```python
from build123d import *

# Parameters (mm, degrees)
SKETCH1_R           = 3.175
BOSS_EXTRUDE1_DEPTH = 57.15


with BuildPart() as part:
    # Sketch1 → Boss-Extrude1 (new body)
    with BuildSketch(Plane.XZ.offset(57.15)):
        with BuildLine():
            Line((-4.682174209, -4.59023638), (-3.666174209, -6.35))
            Line((-3.666174209, -6.35), (-1.634174209, -6.35))
            ThreePointArc((-1.634174209, -6.35), (0, -4.715825791), (1.634174209, -6.35))
            Line((1.634174209, -6.35), (3.666174209, -6.35))
            Line((3.666174209, -6.35), (4.682174209, -4.59023638))
            ThreePointArc((4.682174209, -4.59023638), (4.084024935, -2.357912895), (6.316348419, -1.75976362))
            Line((6.316348419, -1.75976362), (7.332348419, 0))
            Line((7.332348419, 0), (6.316348419, 1.75976362))
            ThreePointArc((6.316348419, 1.75976362), (4.084024935, 2.357912895), (4.682174209, 4.59023638))
            Line((4.682174209, 4.59023638), (3.666174209, 6.35))
            Line((3.666174209, 6.35), (1.634174209, 6.35))
            ThreePointArc((1.634174209, 6.35), (0, 4.715825791), (-1.634174209, 6.35))
            Line((-1.634174209, 6.35), (-3.666174209, 6.35))
            Line((-3.666174209, 6.35), (-4.682174209, 4.59023638))
            ThreePointArc((-4.682174209, 4.59023638), (-4.084024935, 2.357912895), (-6.316348419, 1.75976362))
            Line((-6.316348419, 1.75976362), (-7.332348419, 0))
            Line((-7.332348419, 0), (-6.316348419, -1.75976362))
            ThreePointArc((-6.316348419, -1.75976362), (-4.084024935, -2.357912895), (-4.682174209, -4.59023638))
        make_face()
        Circle(SKETCH1_R, mode=Mode.SUBTRACT)
    extrude(amount=-BOSS_EXTRUDE1_DEPTH)


solid = part.part
```
Could you check a few things on this model? Use its own coordinates, in mm. Round coordinates to 2 decimals unless told otherwise and drop trailing zeros. Order: outer loops, then holes, each group sorted by start corner. A loop starts at its lowest first (then second) coordinate and runs counter-clockwise, first axis right, second up. Notation, with made-up numbers: (23.25, -30.75) -> (33.25, -30.75) arc R10 cw to (33.25, -17.75) -> close; hole circle Ø3 at (77.5, -2.5). An arc over 180 degrees is marked (long way). One line per question, with ' | ' between items.
Q1. If we section it at A-A on x = 0: Write out the boundary of the cut face in (y, z) (3 decimals).
Computed values:
outline: (-57.15, -4.716) -> (0, -4.716) -> (0, -3.175) -> (-57.15, -3.175) -> close; (-57.15, 3.175) -> (0, 3.175) -> (0, 4.716) -> (-57.15, 4.716) -> close
Q2. We'd pull the mould along X, two halves only. Please class faces 1 (the face through (-0.036, -28.975, -4.716)), 2 (the face through (6.83, -28.98, 0.87)), 3 (the face through (2, 0, 3)): released by +X, released by -X, zero draft, split by the parting line, or undercut.
Computed values:
face 1: undercut | face 2: released by +X | face 3: zero draft
Q3. If we section it at C-C on z = 2.25: Write out the boundary of the cut face in (x, y), plus the area to 3 significant figures.
Computed values:
outline: (-4.15, -57.15) -> (-2.24, -57.15) -> (-2.24, 0) -> (-4.15, 0) -> close; (2.24, -57.15) -> (4.15, -57.15) -> (4.15, 0) -> (2.24, 0) -> close | area: 219 mm²
Q4. If I drill on line 1 (Z direction, x = 0, y = -12.5) (3 decimals); line 2 (Z direction, x = 2.5, y = -26.5); line 3 (X direction, y = -49.5, z = 0.5), over which ranges is the centre line in solid material (lowest first)? Write a range as from..to.
Computed values:
line 1: -4.716..-3.175, 3.175..4.716 | line 2: -6.35..-1.96, 1.96..6.35 | line 3: -7.04..-3.14, 3.14..7.04
Q5. I'm going to push flat-ended pins straight in: pin 1 (1.5 mm diameter, centred on y = -26, z = -1.5, fed in from -X); pin 2 (1 mm diameter, centred on x = 0, y = -29, fed in from -Z); pin 3 (5 mm diameter, centred on x = 0, z = 0, fed in from +Y). Where does each tip first touch, or does it pass through?
Computed values:
pin 1: x = -6.9 | pin 2: z = -4.79 | pin 3: through
Q6. If we section it at B-B on y = -6: Write out the boundary of the cut face in (x, z) (3 decimals), plus the area to 3 significant figures.
Computed values:
outline: (-7.332, 0) -> (-6.316, -1.76) arc R1.634 cw to (-4.682, -4.59) -> (-3.666, -6.35) -> (-1.634, -6.35) arc R1.634 cw to (1.634, -6.35) -> (3.666, -6.35) -> (4.682, -4.59) arc R1.634 cw to (6.316, -1.76) -> (7.332, 0) -> (6.316, 1.76) arc R1.634 cw to (4.682, 4.59) -> (3.666, 6.35) -> (1.634, 6.35) arc R1.634 cw to (-1.634, 6.35) -> (-3.666, 6.35) -> (-4.682, 4.59) arc R1.634 cw to (-6.316, 1.76) -> close; hole circle Ø6.35 at (0, 0) | area: 82.8 mm²
